from build123d import *

# Parameters (mm, degrees)
BOSS_EXTRUDE1_DEPTH      = 4
BOSS_EXTRUDE1_DEPTH_BACK = 4
BOSS_EXTRUDE2_DEPTH      = 2.5
CHAMFER1_SIZE            = 1
CUT_EXTRUDE1_DEPTH       = 8.5
CHAMFER2_SIZE            = 0.5


with BuildPart() as part:
    # Sketch1 → Boss-Extrude1 (new, two sides: drawn at the far end of the back side and taken through both)
    with BuildSketch(Plane.YZ.offset(-BOSS_EXTRUDE1_DEPTH_BACK)):
        Polygon((-3.3, 9.2), (3.3, 9.2), (6.6, 5.2), (6.6, 4.2), (3.3, 4.2), (3.3, 0), (3.3, -1), (5.55, -3.25), (3.3, -5.5), (5.55, -7.75), (3.3, -10), (-3.3, -10), (-5.55, -7.75), (-3.3, -5.5), (-5.55, -3.25), (-3.3, -1), (-3.3, 0), (-3.3, 4.2), (-6.6, 4.2), (-6.6, 5.2), align=None)
    extrude(amount=BOSS_EXTRUDE1_DEPTH + BOSS_EXTRUDE1_DEPTH_BACK)

    # Sketch2 → Boss-Extrude2 (add)
    with BuildSketch(Plane.YZ.offset(4)):
        Polygon((-3.3, 0), (3.3, 0), (3.3, -1), (5.55, -3.25), (3.3, -5.5), (5.55, -7.75), (3.3, -10), (-3.3, -10), (-5.55, -7.75), (-3.3, -5.5), (-5.55, -3.25), (-3.3, -1), align=None)
    extrude(amount=BOSS_EXTRUDE2_DEPTH)

    # Chamfer1
    chamfer1_edges = [part.edges().sort_by_distance(p)[0] for p in [
        (-4, -4.95, 7.2),
        (-4, -6.6, 4.7),
        (-4, 4.95, 7.2),
        (4, 4.95, 7.2),
        (4, 0, 9.2),
        (4, -4.95, 7.2),
        (4, -6.6, 4.7),
        (4, 6.6, 4.7),
        (-4, 6.6, 4.7),
        (-4, 0, 9.2),
    ]]
    chamfer(chamfer1_edges, length=CHAMFER1_SIZE)

    # Sketch3 → Cut-Extrude1 (cut)
    with BuildSketch(Plane(origin=(-4, 0, 0), x_dir=(0, -1, 0), z_dir=(-1, 0, 0))):
        Polygon((0, -8), (2, -10), (-2, -10), align=None)
    extrude(amount=-CUT_EXTRUDE1_DEPTH, mode=Mode.SUBTRACT)

    # Chamfer2
    chamfer2_edges = [part.edges().sort_by_distance(p)[0] for p in [
        (-4, 2.65, -10),
        (-4, 1, -9),
        (-4, -1, -9),
        (-4, -3.3, 1.6),
        (-4, -4.425, -2.125),
        (-4, -4.425, -4.375),
        (-4, -4.425, -6.625),
        (-4, -4.425, -8.875),
        (-4, -2.65, -10),
        (-4, 4.425, -8.875),
        (-4, 4.425, -6.625),
        (-4, 4.425, -4.375),
        (-4, 4.425, -2.125),
        (-4, 3.3, 1.6),
    ]]
    chamfer(chamfer2_edges, length=CHAMFER2_SIZE)


solid = part.part
Build history of the part. All positions in model axes, mm. A direction names the side the tool comes from. Coordinates: 2 decimals unless noted, no trailing zeros. Order: outer loops, then holes, each group sorted by start corner. A loop starts at its lowest first (then second) coordinate and runs counter-clockwise, first axis right, second up. Notation, with made-up numbers: (-12.5, 62) - (-4.5, 62) arc R24 cw to (-4.5, 95) - close; hole circle Ø1 at (16.5, -39). An arc over 180 degrees is marked (long way). Write item = value, one per line. Start each with the question number.
1) Saw through at C-C on y = -1. Write the cut outline in (x, z), then the cut area to 3 significant figures.
2) 3-axis set-ups, long thin cutter, end or side, ignore diameter. For faces 1 (the face through (1.4, 4.4, -2.1)), 2 (the face through (1.4, -4.4, -4.4)), 3 (the face through (0, 1, -9)), 4 (the face through (4, 0, 4)): which of +Z, -Z, +X, -X, +Y, -Y reach the whole face in a straight line?
3) Saw through at B-B on x = 5.5. Write the cut outline in (y, z), then the cut area to 4 significant figures.
4) Flat gauge pins, fed straight in: pin 1 Ø4 at (x, z) = (2, 0.5) entering from +Y; pin 2 Ø1 at (x, z) = (-1.5, -6) entering from +Y; pin 3 Ø1.6 at (y, z) = (1, -9.5) entering from -X. Where does each tip first touch, or does it go through?
5) Saw through at D-D on z = 6. Write the cut outline in (x, y), then the cut area to 3 significant figures.
6) Saw through at A-A on y = 4. Write the cut outline in (x, z), then the cut area to 3 significant figures.
7) Wall check: line 1 along Z through (x, y) = (-1.75, 4); line 2 along Z through (x, y) = (-2.5, 3.5); line 3 along X through (y, z) = (-1.25, 5). Give the ranges that are in metal, low to high. Write a range as from..to.
From the geometry:
q1.outline = (-4, -8.29) - (-3.5, -9) - (4.5, -9) - (4.5, -10) - (6.5, -10) - (6.5, 0) - (4, 0) - (4, 8.2) - (3, 9.2) - (-3, 9.2) - (-4, 8.2) - close
q1.area = 169 mm^2
q2.face_1 = +X, -X, +Y
q2.face_2 = +X, -X, -Y
q2.face_3 = -Z, -X
q2.face_4 = +Z, +X, +Y, -Y
q3.outline = (-5.55, -7.75) - (-3.3, -10) - (3.3, -10) - (5.55, -7.75) - (3.3, -5.5) - (5.55, -3.25) - (3.3, -1) - (3.3, 0) - (-3.3, 0) - (-3.3, -1) - (-5.55, -3.25) - (-3.3, -5.5) - close
q3.area = 86.25 mm^2
q4.pin_1 = 3.8
q4.pin_2 = 4.3
q4.pin_3 = -3.95
q5.outline = (-4, -4.64) - (-3, -5.94) - (3, -5.94) - (4, -4.64) - (4, 4.64) - (3, 5.94) - (-3, 5.94) - (-4, 4.64) - close
q5.area = 92.4 mm^2
q6.outline = (-4, -8.59) - (-3.5, -9.3) - (6.5, -9.3) - (6.5, -6.2) - (-3.5, -6.2) - (-4, -6.91) - close; (-4, -4.09) - (-3.5, -4.8) - (6.5, -4.8) - (6.5, -1.7) - (-3.5, -1.7) - (-4, -2.41) - close; (-4, 4.2) - (4, 4.2) - (4, 6.78) - (3, 8.35) - (-3, 8.35) - (-4, 6.78) - close
q6.area = 96.0 mm^2
q7.line_1 = -9.3..-6.2, -4.8..-1.7, 4.2..8.35
q7.line_2 = -9.8..-5.7, -5.3..-1.2, 4.2..8.96
q7.line_3 = -4..4
